from build123d import *
from OCP.BRepFilletAPI import BRepFilletAPI_MakeChamfer

# Parameters (mm, degrees)
SKETCH4_W                = 12.46
SKETCH4_H                = 17.25
BOSS_EXTRUDE3_DEPTH      = 6
BOSS_EXTRUDE6_DEPTH      = 7.3
BOSS_EXTRUDE6_DEPTH_BACK = 17.25
SKETCH8_R                = 12.546781182
SKETCH8_R_2              = 11.15
BOSS_EXTRUDE4_DEPTH      = 17.25
SKETCH6_R                = 2
CUT_EXTRUDE1_DEPTH       = 5
CHAMFER1_SIZE            = 0.5
CHAMFER1_SIZE_2          = 0.866025404
SKETCH10_W               = 12.46
SKETCH10_H               = 23.7
CUT_EXTRUDE3_DEPTH       = 17.25
CUT_EXTRUDE4_REACH       = 43.938
SKETCH11_W               = 5
SKETCH11_H               = 3
BOSS_EXTRUDE7_START      = -7.3
BOSS_EXTRUDE7_DEPTH      = 7.3
BOSS_EXTRUDE9_START      = 10
BOSS_EXTRUDE9_DEPTH      = 10
BOSS_EXTRUDE10_DEPTH     = 25.093562364
SKETCH18_W               = 20
SKETCH18_H               = 12.438292938
CUT_EXTRUDE5_DEPTH       = 2
CUT_EXTRUDE6_DEPTH       = 57.41497434
CUT_EXTRUDE6_DEPTH_BACK  = 57.41497434
SKETCH19_R               = 1.25
FILLET1_R                = 10
CUT_EXTRUDE7_DEPTH       = 55.620050849
CUT_EXTRUDE7_DEPTH_BACK  = 55.620050849
SKETCH20_W               = 25.093562364
SKETCH20_H               = 36.096781182
BOSS_EXTRUDE11_DEPTH     = 43.5
CUT_EXTRUDE8_DEPTH       = 40.12140358
CUT_EXTRUDE8_DEPTH_BACK  = 40.12140358
CUT_EXTRUDE9_DEPTH       = 40.12140358
CUT_EXTRUDE9_DEPTH_BACK  = 40.12140358


with BuildPart() as part:
    # Sketch4 → Boss-Extrude3 (new body)
    with BuildSketch(Plane.XY):
        with Locations((0, -1.35)):
            Rectangle(SKETCH4_W, SKETCH4_H)
    extrude(amount=BOSS_EXTRUDE3_DEPTH)



with BuildPart() as body_2:
    # Sketch8 → Boss-Extrude6 (new, two sides: drawn at the far end of the back side and taken through both)
    with BuildSketch(Plane(origin=(0, -9.975, 0), x_dir=(-1, 0, 0), z_dir=(0, -1, 0)).offset(-BOSS_EXTRUDE6_DEPTH_BACK)):
        with Locations(Location((0, -23.55, 0), (0, 0, 90))):
            Circle(SKETCH8_R)
        with Locations(Location((0, -23.55, 0), (0, 0, 90))):
            Circle(SKETCH8_R_2, mode=Mode.SUBTRACT)
    extrude(amount=BOSS_EXTRUDE6_DEPTH + BOSS_EXTRUDE6_DEPTH_BACK)


with BuildPart() as part_1:
    add(part.part)

    add(body_2.part)  # Boss-Extrude4 merges body 2
    # Sketch5 → Boss-Extrude4 (add)
    with BuildSketch(Plane(origin=(0, 7.275, 0), x_dir=(1, 0, 0), z_dir=(0, 1, 0))):
        with BuildLine():
            Line((12.546781182, -23.55), (12.546781182, 0))
            Line((12.546781182, 0), (6.23, 0))
            Line((6.23, 0), (6.23, -29.7))
            Line((6.23, -29.7), (-6.23, -29.7))
            Line((-6.23, -29.7), (-6.23, 0))
            Line((-6.23, 0), (-12.546781182, 0))
            Line((-12.546781182, 0), (-12.546781182, -23.55))
            ThreePointArc((-12.546781182, -23.55), (0, -36.096781182), (12.546781182, -23.55))
        make_face()
    extrude(amount=-BOSS_EXTRUDE4_DEPTH)

    # Sketch6 → Cut-Extrude1 (cut)
    with BuildSketch(Plane(origin=(0, 7.275, 0), x_dir=(1, 0, 0), z_dir=(0, 1, 0))):
        with Locations(Location((0, -3.5, 0), (0, 0, 270))):
            Circle(SKETCH6_R)
        with Locations(Location((0, -32.2, 0), (0, 0, 270))):
            Circle(SKETCH6_R)
    extrude(amount=-CUT_EXTRUDE1_DEPTH, mode=Mode.SUBTRACT)

    # Chamfer1
    chamfer1_edges_1 = [part_1.edges().sort_by_distance(p)[0] for p in [
        (0, 7.275, 1.5),
    ]]
    chamfer1_side_1 = [part_1.faces().sort_by_distance(p)[0] for p in [
        (0, 7.275, 1.49),
    ]]
    chamfer1_edges_2 = [part_1.edges().sort_by_distance(p)[0] for p in [
        (0, 7.275, 30.2),
    ]]
    chamfer1_side_2 = [part_1.faces().sort_by_distance(p)[0] for p in [
        (0, 7.275, 30.19),
    ]]
    chamfer1 = BRepFilletAPI_MakeChamfer(part_1.part.solid().wrapped)
    for e in chamfer1_edges_1:
        chamfer1.Add(CHAMFER1_SIZE - 0.0001, CHAMFER1_SIZE_2 - 0.0001, e.wrapped, chamfer1_side_1[0].wrapped)
    for e in chamfer1_edges_2:
        chamfer1.Add(CHAMFER1_SIZE - 0.0001, CHAMFER1_SIZE_2 - 0.0001, e.wrapped, chamfer1_side_2[0].wrapped)
    add(Compound.cast(chamfer1.Shape()), mode=Mode.REPLACE)  # a hair under: the kernel refuses the full size

    # Sketch10 → Cut-Extrude3 (cut)
    with BuildSketch(Plane(origin=(0, 7.275, 0), x_dir=(1, 0, 0), z_dir=(0, 1, 0))):
        with Locations((0, -17.85)):
            Rectangle(SKETCH10_W, SKETCH10_H)
    extrude(amount=-CUT_EXTRUDE3_DEPTH, mode=Mode.SUBTRACT)

    # Sketch11 → Cut-Extrude4 (cut, up to next)
    with BuildSketch(Plane.XY.offset(36.096781182), mode=Mode.PRIVATE) as cut_extrude4_sk1:
        with Locations((0, -8.475)):
            Rectangle(SKETCH11_W, SKETCH11_H)
    cut_extrude4_tool1 = extrude(cut_extrude4_sk1.sketch, amount=-CUT_EXTRUDE4_REACH, mode=Mode.PRIVATE) & part_1.part
    add(cut_extrude4_tool1.solids().sort_by_distance((0, -8.475, 36.096781))[0], mode=Mode.SUBTRACT)

    # Sketch13 → Boss-Extrude7 (add)
    with BuildSketch(Plane.XZ.offset(17.275).offset(BOSS_EXTRUDE7_START)):
        with BuildLine():
            Line((-12.546781182, 23.55), (-12.546781182, 0))
            Line((-12.546781182, 0), (12.546781182, 0))
            Line((12.546781182, 0), (12.546781182, 23.55))
            ThreePointArc((12.546781182, 23.55), (0, 11.003218818), (-12.546781182, 23.55))
        make_face()
    extrude(amount=BOSS_EXTRUDE7_DEPTH)

    # Sketch15 → Boss-Extrude9 (add)
    with BuildSketch(Plane(origin=(0, 7.275, 0), x_dir=(1, 0, 0), z_dir=(0, 1, 0)).offset(BOSS_EXTRUDE9_START)):
        with BuildLine():
            Line((-12.546781182, 0), (12.546781182, 0))
            Line((12.546781182, 0), (12.546781182, -23.55))
            ThreePointArc((12.546781182, -23.55), (0, -36.096781182), (-12.546781182, -23.55))
            Line((-12.546781182, -23.55), (-12.546781182, 0))
        make_face()
        with BuildLine():
            Line((-6.23, -0.8), (6.23, -0.8))
            Line((6.23, -0.8), (6.23, -33.5))
            ThreePointArc((6.23, -33.5), (5.937106781, -34.207106781), (5.23, -34.5))
            Line((5.23, -34.5), (-5.23, -34.5))
            ThreePointArc((-5.23, -34.5), (-5.937106781, -34.207106781), (-6.23, -33.5))
            Line((-6.23, -33.5), (-6.23, -0.8))
        make_face(mode=Mode.SUBTRACT)
    extrude(amount=-BOSS_EXTRUDE9_DEPTH)

    # Sketch17 → Boss-Extrude10 (add)
    with BuildSketch(Plane(origin=(-12.546781182, 4.728218818, 0), x_dir=(0, -1, 0), z_dir=(1, 0, 0))):
        Polygon((26.478218818, 25), (26.478218818, 0), (-17.021781182, 0), (-17.021781182, 25), (-13.021781182, 25), (-13.021781182, 5), (22.478218818, 5), (22.478218818, 25), align=None)
    extrude(amount=BOSS_EXTRUDE10_DEPTH)

    # Sketch18 → Cut-Extrude5 (cut)
    with BuildSketch(Plane.ZX.offset(-17.75)):
        with Locations((-15, 0)):
            Rectangle(SKETCH18_W, SKETCH18_H)
    extrude(amount=-CUT_EXTRUDE5_DEPTH, mode=Mode.SUBTRACT)

    # Sketch19 → Cut-Extrude6 (cut, two sides: drawn at the far end of the back side and taken through both)
    with BuildSketch(Plane.ZX.offset(-19.75).offset(-CUT_EXTRUDE6_DEPTH_BACK)):
        with Locations((-20, 0)):
            Circle(SKETCH19_R)
    extrude(amount=CUT_EXTRUDE6_DEPTH + CUT_EXTRUDE6_DEPTH_BACK, mode=Mode.SUBTRACT)

    # Fillet1
    fillet1_edges = [part_1.edges().sort_by_distance(p)[0] for p in [
        (12.546781182, -19.75, -25),
        (-12.546781182, -19.75, -25),
        (-12.546781182, 19.75, -25),
        (12.546781182, 19.75, -25),
    ]]
    fillet(fillet1_edges, radius=FILLET1_R)

    # Sketch20 → Cut-Extrude7 (cut, two sides: drawn at the far end of the back side and taken through both)
    with BuildSketch(Plane(origin=(0, 17.275, 0), x_dir=(1, 0, 0), z_dir=(0, 1, 0)).offset(-CUT_EXTRUDE7_DEPTH_BACK)):
        with Locations((0, -18.048390591)):
            Rectangle(SKETCH20_W, SKETCH20_H)
    extrude(amount=CUT_EXTRUDE7_DEPTH + CUT_EXTRUDE7_DEPTH_BACK, mode=Mode.SUBTRACT)

    # Sketch21 → Boss-Extrude11 (add)
    with BuildSketch(Plane(origin=(0, 21.75, 0), x_dir=(1, 0, 0), z_dir=(0, 1, 0))):
        Polygon((12.546781182, 0), (-0.025415104, -30), (-12.546781182, 0), align=None)
    extrude(amount=-BOSS_EXTRUDE11_DEPTH)

    # Sketch22 → Cut-Extrude8 (cut, two sides: drawn at the far end of the back side and taken through both)
    with BuildSketch(Plane(origin=(0, 0, 0), x_dir=(0, 0, -1), z_dir=(1, 0, 0)).offset(-CUT_EXTRUDE8_DEPTH_BACK)):
        Polygon((0, 21.75), (-30, 0.01), (-30, 21.75), align=None)
        Polygon((0, -21.75), (-30, -21.75), (-30, -0.01), align=None)
    extrude(amount=CUT_EXTRUDE8_DEPTH + CUT_EXTRUDE8_DEPTH_BACK, mode=Mode.SUBTRACT)

    # Sketch23 → Cut-Extrude9 (cut, two sides: drawn at the far end of the back side and taken through both)
    with BuildSketch(Plane(origin=(0, 0, 0), x_dir=(-1, 0, 0), z_dir=(0, 0, -1)).offset(-CUT_EXTRUDE9_DEPTH_BACK)):
        Polygon((12.546781182, 17.75), (0, 0), (12.546781182, -21.75), align=None)
    extrude(amount=CUT_EXTRUDE9_DEPTH + CUT_EXTRUDE9_DEPTH_BACK, mode=Mode.SUBTRACT)


solid = part_1.part
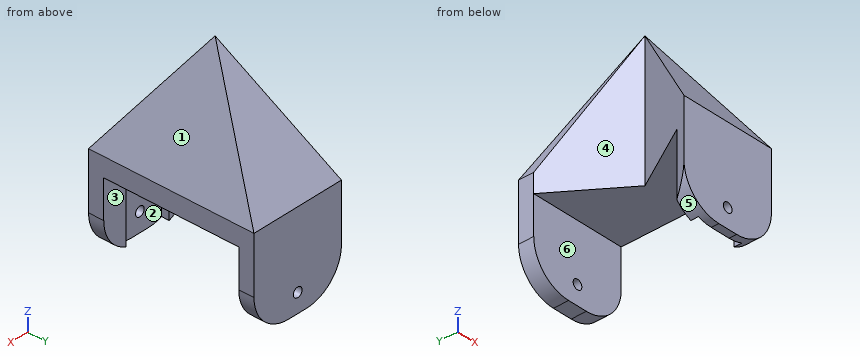
CAD build for the part. Positions are in the model's coordinates, mm. Face numbers are marked on the shaded views. A direction names the side the tool comes from. Coordinates: 2 decimals unless noted, no trailing zeros. Loops run counter-clockwise (first coordinate to the right, second up) from the corner with the lowest first, then second, coordinate; pieces in that order, holes last. Notation, with made-up numbers: (-4.5, -10.75) - (11.5, -10.75) arc R19 ccw to (11.5, 21.25) - close; hole circle Ø10 at (55, -37). An arc over 180 degrees is marked (long way). Use one line per item in the form item = value. Start each with the question number.
1) Flat gauge pins, fed straight in: pin 1 (3 mm diameter, centred on x = 3, y = -4.5, fed in from +Z); pin 2 (6 mm diameter, centred on x = -0.5, z = 9.5, fed in from +Y); pin 3 (1 mm diameter, centred on x = -4, z = 1, fed in from -Y). Where does each tip first touch, or does it go through?
2) Band-saw the part on C-C (x = 9). Give the cut face in (y, z).
3) Band-saw the part on A-A (z = -6.5). Give the cut face in (x, y).
4) Tool access for the marked faces 4, 5 and 6: list every direction of +Z, -Z, +X, -X, +Y, -Y with a clear straight run to the whole face (end or side of a thin tool).
5) Drill centre lines: L1, parallel to Y at x = -7.25, z = -15.5; L2, parallel to Y at x = -3.75, z = -6; L3, parallel to X at y = -20, z = -20. Where is each one in solid material? Low to high. Write a range as from..to.
6) Two-plate mould, pull along X, no slides. Class the marked faces 1, 2 and 3: +X half, -X half, draft (parallel to the pull), parting line (faces both ways), or undercut.
7) Band-saw the part on D-D (y = -2). Give the cut face in (x, z).
8) Band-saw the part on B-B (z = -20). Give the cut face in (x, y), and give its area (3 significant figures).
Check values:
q1.pin_1 = 25.28
q1.pin_2 = 17.04
q1.pin_3 = -21.39
q2.outline = (-21.75, -22.64) - (-17.75, -22.64) - (-17.75, -5) - (17.75, -5) - (17.75, -22.64) - (21.75, -22.64) - (21.75, 0) - (15.62, 8.46) - (-15.62, 8.46) - (-21.75, 0) - close
q3.outline = (-12.55, -21.75) - (12.55, -21.75) - (12.55, -17.75) - (6.22, -17.75) - (6.22, -19.75) - (-6.22, -19.75) - (-6.22, -17.75) - (-10.24, -17.75) - close; (-12.55, 17.75) - (12.55, 17.75) - (12.55, 21.75) - (-12.55, 21.75) - close
q4.face_4 = +Z, -Z, -X
q4.face_5 = -Z, -X, +Y, -Y
q4.face_6 = -Z, +X, -X
q5.L1 = -21.75..-17.75, 17.75..21.75
q5.L2 = -21.75..-19.75, 17.75..21.75
q5.L3 = -11.21..-1.25, 1.25..11.21
q6.face_1 = +X half
q6.face_2 = undercut
q6.face_3 = draft
q7.outline = (-1.15, -5) - (12.55, -5) - (12.55, 0) - (1.13, 27.25) - (-1.15, 27.25) - close
q8.outline = (-11.21, -21.75) - (-1.25, -21.75) - (-1.25, -19.75) - (-6.22, -19.75) - (-6.22, -17.75) - (-10.24, -17.75) - (-11.21, -19.43) - close; (-11.21, 17.75) - (-1.25, 17.75) - (-1.25, 21.75) - (-11.21, 21.75) - close; (1.25, -21.75) - (11.21, -21.75) - (11.21, -17.75) - (6.22, -17.75) - (6.22, -19.75) - (1.25, -19.75) - close; (1.25, 17.75) - (11.21, 17.75) - (11.21, 21.75) - (1.25, 21.75) - close
q8.area = 139 mm2
